Check sheet for the drawn part. Datum: minimum x, y, z corner. Units: mm. A direction names the side the tool comes from. Round coordinates to 2 decimals unless told otherwise and drop trailing zeros. Order: outer loops, then holes, each group sorted by start corner. A loop starts at its lowest first (then second) coordinate and runs counter-clockwise, first axis right, second up.
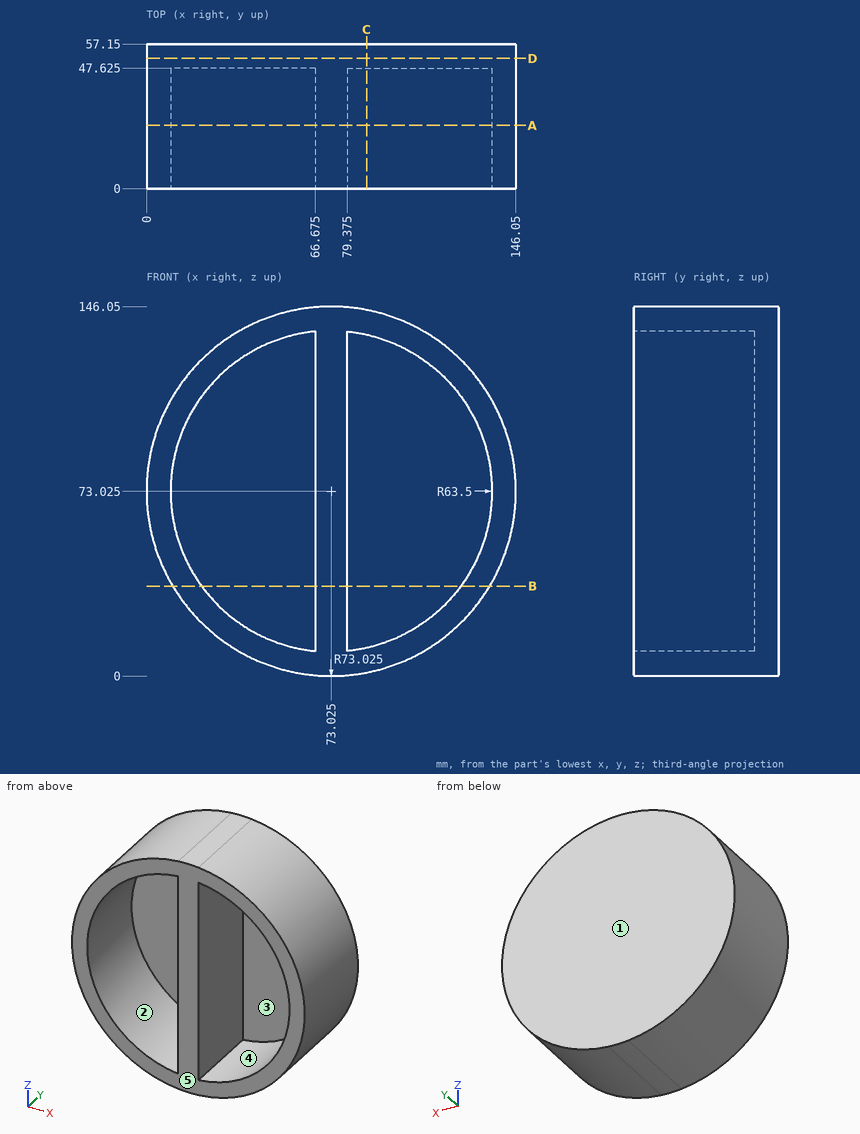
1) Sectioned sample at D-D on y = 51.5. Record the cut outline in (x, z) (3 decimals).
2) Sectioned sample at A-A on y = 25. Record the cut outline in (x, z) (3 decimals), and give its area (3 significant figures).
3) Set-up check for the marked faces 4 and 5: record each of +Z, -Z, +X, -X, +Y, -Y from which the full face is reachable in a straight line by a thin tool's end or side.
4) Gauge pin test, flat ends, axial feed: pin 1 (24 mm diameter, centred on y = 16, z = 49.5, fed in from +X); pin 2 (5 mm diameter, centred on x = 111.5, z = 111.5, fed in from -Y) (3 decimals); pin 3 (24 mm diameter, centred on y = 16.5, z = 102.5, fed in from -X). Record the tip position at first contact, or that the pin passes through.
5) Sectioned sample at C-C on x = 87. Record the cut outline in (y, z) (3 decimals).
6) Sectioned sample at B-B on z = 35.5. Record the cut outline in (x, y) (3 decimals).
7) Scan lines: line 1 (Z direction, x = 79.5, y = 12.5); line 2 (X direction, y = 9, z = 22) (3 decimals); line 3 (X direction, y = 30, z = 66) (3 decimals). Record each from-to range of solid material in increasing order.
8) Draft check along X on the marked faces 1, 2 and 3. Enter one of: pulls with the +X half, pulls with the -X half, needs draft (parallel to the pull), parting line crosses it, or undercut.
Values found:
1. outline: circle Ø146.05 at (73.025, 73.025)
2. outline: circle Ø146.05 at (73.025, 73.025); hole (66.675, 9.843) - (66.675, 136.207) arc R63.5 ccw to start; hole (79.375, 9.843) arc R63.5 ccw to (79.375, 136.207) - close
2. area: 5,700 mm2
3. face 4: -Y
3. face 5: +Z, -Z, +X, -X, -Y
4. pin 1: stops at x = 145.13
4. pin 2: stops at y = 47.625
4. pin 3: stops at x = 2.12
5. outline: (0, 1.35) - (57.15, 1.35) - (57.15, 144.7) - (0, 144.7) - (0, 134.968) - (47.625, 134.968) - (47.625, 11.082) - (0, 11.082) - close
6. outline: (10.379, 0) - (21.799, 0) - (21.799, 47.625) - (66.675, 47.625) - (66.675, 0) - (79.375, 0) - (79.375, 47.625) - (124.251, 47.625) - (124.251, 0) - (135.671, 0) - (135.671, 57.15) - (10.379, 57.15) - close
7. line 1: z = 0.29 to 9.86, 136.19 to 145.76
7. line 2: x = 20.784 to 35.227, 66.675 to 79.375, 110.823 to 125.266
7. line 3: x = 0.339 to 9.915, 66.675 to 79.375, 136.135 to 145.711
8. face 1: needs draft
8. face 2: undercut
8. face 3: undercut
